```python
from build123d import *

# Parameters (mm, degrees)
SKETCH_1_W          = 60
SKETCH_1_H          = 17
EXTRUDE_1_DEPTH     = 1.2
CUT_EXTRUDE_1_REACH = 33.204
SKETCH_4_R          = 3.25
SKETCH_4_W          = 9.6
SKETCH_4_H          = 3.4
SKETCH_4_W_2        = 7
SKETCH_4_H_2        = 3.5
SKETCH_4_W_3        = 8
SKETCH_4_H_3        = 2.9
SKETCH_4_W_4        = 6.5
FILLET_2_R          = 1
CHAMFER_1_SIZE      = 0.6
SKETCH_5_W          = 1.5
SKETCH_5_H          = 8
EXTRUDE_2_DEPTH     = 1.2
SKETCH_6_W          = 28.5
SKETCH_6_H          = 1.6
EXTRUDE_3_DEPTH     = 4
FILLET_3_R          = 1
CHAMFER_2_SIZE      = 1
CHAMFER_4_SIZE      = 1
FILLET_4_R          = 2
CHAMFER_5_SIZE      = 0.4


with BuildPart() as part:
    # 草图1 → 凸台-拉伸1 (new body)
    with BuildSketch(Plane(origin=(0, 0, 0), x_dir=(1, 0, 0), z_dir=(0, 1, 0))):
        Rectangle(SKETCH_1_W, SKETCH_1_H)
    extrude(amount=EXTRUDE_1_DEPTH)

    # 草图4 → 切除-拉伸1 (cut, up to next)
    with BuildSketch(Plane(origin=(0, 1.2, 0), x_dir=(1, 0, 0), z_dir=(0, 1, 0)), mode=Mode.PRIVATE) as cut_extrude_1_sk1:
        with Locations(Location((22.298485985, 3.98318929, 0), (0, 0, 270))):
            Circle(SKETCH_4_R)
    cut_extrude_1_tool1 = extrude(cut_extrude_1_sk1.sketch, amount=-CUT_EXTRUDE_1_REACH, mode=Mode.PRIVATE) & part.part
    # 草图4 → 切除-拉伸1 (cut, up to next)
    with BuildSketch(Plane(origin=(0, 1.2, 0), x_dir=(1, 0, 0), z_dir=(0, 1, 0)), mode=Mode.PRIVATE) as cut_extrude_1_sk2:
        with Locations((-20.471722325, 2.6)):
            Rectangle(SKETCH_4_W, SKETCH_4_H)
    cut_extrude_1_tool2 = extrude(cut_extrude_1_sk2.sketch, amount=-CUT_EXTRUDE_1_REACH, mode=Mode.PRIVATE) & part.part
    # 草图4 → 切除-拉伸1 (cut, up to next)
    with BuildSketch(Plane(origin=(0, 1.2, 0), x_dir=(1, 0, 0), z_dir=(0, 1, 0)), mode=Mode.PRIVATE) as cut_extrude_1_sk3:
        with Locations((-5.682926277, 2.55)):
            Rectangle(SKETCH_4_W_2, SKETCH_4_H_2)
    cut_extrude_1_tool3 = extrude(cut_extrude_1_sk3.sketch, amount=-CUT_EXTRUDE_1_REACH, mode=Mode.PRIVATE) & part.part
    # 草图4 → 切除-拉伸1 (cut, up to next)
    with BuildSketch(Plane(origin=(0, 1.2, 0), x_dir=(1, 0, 0), z_dir=(0, 1, 0)), mode=Mode.PRIVATE) as cut_extrude_1_sk4:
        with Locations((7.788485985, 2.55)):
            Rectangle(SKETCH_4_W_2, SKETCH_4_H_2)
    cut_extrude_1_tool4 = extrude(cut_extrude_1_sk4.sketch, amount=-CUT_EXTRUDE_1_REACH, mode=Mode.PRIVATE) & part.part
    # 草图4 → 切除-拉伸1 (cut, up to next)
    with BuildSketch(Plane(origin=(0, 1.2, 0), x_dir=(1, 0, 0), z_dir=(0, 1, 0)), mode=Mode.PRIVATE) as cut_extrude_1_sk5:
        with Locations((21.05, -4.584803861)):
            Rectangle(SKETCH_4_W_3, SKETCH_4_H_3)
    cut_extrude_1_tool5 = extrude(cut_extrude_1_sk5.sketch, amount=-CUT_EXTRUDE_1_REACH, mode=Mode.PRIVATE) & part.part
    # 草图4 → 切除-拉伸1 (cut, up to next)
    with BuildSketch(Plane(origin=(0, 1.2, 0), x_dir=(1, 0, 0), z_dir=(0, 1, 0)), mode=Mode.PRIVATE) as cut_extrude_1_sk6:
        with Locations((-1.65, -4.884803861)):
            Rectangle(SKETCH_4_W_4, SKETCH_4_H_2)
    cut_extrude_1_tool6 = extrude(cut_extrude_1_sk6.sketch, amount=-CUT_EXTRUDE_1_REACH, mode=Mode.PRIVATE) & part.part
    # 草图4 → 切除-拉伸1 (cut, up to next)
    with BuildSketch(Plane(origin=(0, 1.2, 0), x_dir=(1, 0, 0), z_dir=(0, 1, 0)), mode=Mode.PRIVATE) as cut_extrude_1_sk7:
        with Locations((-10.15, -4.884803861)):
            Rectangle(SKETCH_4_W_4, SKETCH_4_H_2)
    cut_extrude_1_tool7 = extrude(cut_extrude_1_sk7.sketch, amount=-CUT_EXTRUDE_1_REACH, mode=Mode.PRIVATE) & part.part
    # 草图4 → 切除-拉伸1 (cut, up to next)
    with BuildSketch(Plane(origin=(0, 1.2, 0), x_dir=(1, 0, 0), z_dir=(0, 1, 0)), mode=Mode.PRIVATE) as cut_extrude_1_sk8:
        with Locations((-20.471722325, -4.834803861)):
            Rectangle(SKETCH_4_W, SKETCH_4_H)
    cut_extrude_1_tool8 = extrude(cut_extrude_1_sk8.sketch, amount=-CUT_EXTRUDE_1_REACH, mode=Mode.PRIVATE) & part.part
    add(cut_extrude_1_tool1.solids().sort_by_distance((22.298486, 1.2, -3.983189))[0], mode=Mode.SUBTRACT)
    add(cut_extrude_1_tool2.solids().sort_by_distance((-20.471722, 1.2, -2.6))[0], mode=Mode.SUBTRACT)
    add(cut_extrude_1_tool3.solids().sort_by_distance((-5.682926, 1.2, -2.55))[0], mode=Mode.SUBTRACT)
    add(cut_extrude_1_tool4.solids().sort_by_distance((7.788486, 1.2, -2.55))[0], mode=Mode.SUBTRACT)
    add(cut_extrude_1_tool5.solids().sort_by_distance((21.05, 1.2, 4.584804))[0], mode=Mode.SUBTRACT)
    add(cut_extrude_1_tool6.solids().sort_by_distance((-1.65, 1.2, 4.884804))[0], mode=Mode.SUBTRACT)
    add(cut_extrude_1_tool7.solids().sort_by_distance((-10.15, 1.2, 4.884804))[0], mode=Mode.SUBTRACT)
    add(cut_extrude_1_tool8.solids().sort_by_distance((-20.471722, 1.2, 4.834804))[0], mode=Mode.SUBTRACT)

    # 圆角2
    fillet_2_edges = [part.edges().sort_by_distance(p)[0] for p in [
        (-9.182926277, 0.6, -4.3),
        (-2.182926277, 0.6, -4.3),
        (4.288485985, 0.6, -4.3),
        (11.288485985, 0.6, -4.3),
        (17.05, 0.6, 6.034803861),
        (25.05, 0.6, 6.034803861),
        (-4.9, 0.6, 6.634803861),
        (-4.9, 0.6, 3.134803861),
        (1.6, 0.6, 3.134803861),
        (1.6, 0.6, 6.634803861),
        (-13.4, 0.6, 6.634803861),
        (-13.4, 0.6, 3.134803861),
        (-6.9, 0.6, 3.134803861),
        (-6.9, 0.6, 6.634803861),
        (-25.271722325, 0.6, 6.534803861),
        (-25.271722325, 0.6, 3.134803861),
        (-15.671722325, 0.6, 3.134803861),
        (-15.671722325, 0.6, 6.534803861),
        (-25.271722325, 0.6, -0.9),
        (-25.271722325, 0.6, -4.3),
        (-15.671722325, 0.6, -4.3),
        (-15.671722325, 0.6, -0.9),
    ]]
    fillet(fillet_2_edges, radius=FILLET_2_R)

    # 倒角1
    chamfer_1_edges = [part.edges().sort_by_distance(p)[0] for p in [
        (-9.182926277, 0.6, -0.8),
        (-2.182926277, 0.6, -0.8),
        (4.288485985, 0.6, -0.8),
        (11.288485985, 0.6, -0.8),
        (17.05, 0.6, 3.134803861),
        (25.05, 0.6, 3.134803861),
    ]]
    chamfer(chamfer_1_edges, length=CHAMFER_1_SIZE)

    # 草图5 → 凸台-拉伸2 (add)
    with BuildSketch(Plane.XZ):
        with Locations((-13.15891381, 0.61681071)):
            Rectangle(SKETCH_5_W, SKETCH_5_H)
        with Locations((13.84108619, 0.61681071)):
            Rectangle(SKETCH_5_W, SKETCH_5_H)
    extrude(amount=EXTRUDE_2_DEPTH)

    # 草图6 → 凸台-拉伸3 (add)
    with BuildSketch(Plane.XZ):
        with Locations((0.34108619, 1.3)):
            Rectangle(SKETCH_6_W, SKETCH_6_H)
    extrude(amount=EXTRUDE_3_DEPTH)

    # 圆角3
    fillet_3_edges = [part.edges().sort_by_distance(p)[0] for p in [
        (-13.90891381, -4, 1.3),
        (14.59108619, -4, 1.3),
    ]]
    fillet(fillet_3_edges, radius=FILLET_3_R)

    # 倒角2
    chamfer_2_edges = [part.edges().sort_by_distance(p)[0] for p in [
        (-13.15891381, -1.2, -3.38318929),
        (-13.15891381, -1.2, 4.61681071),
        (13.84108619, -1.2, -3.38318929),
        (13.84108619, -1.2, 4.61681071),
    ]]
    chamfer(chamfer_2_edges, length=CHAMFER_2_SIZE)

    # 倒角4
    chamfer_4_edges = [part.edges().sort_by_distance(p)[0] for p in [
        (-5.682926277, 0, -4.3),
        (-2.182926277, 0, -2.35),
        (7.788485985, 0, -4.3),
        (11.288485985, 0, -2.35),
        (21.05, 0, 6.034803861),
        (17.05, 0, 4.384803861),
        (-2.475819496, 0, -4.007106781),
        (-8.890033058, 0, -4.007106781),
        (4.581379204, 0, -4.007106781),
        (10.995592766, 0, -4.007106781),
        (24.757106781, 0, 5.741910642),
        (17.342893219, 0, 5.741910642),
        (-5.682926277, 0, -0.8),
        (-9.182926277, 0, -2.35),
        (7.788485985, 0, -0.8),
        (4.288485985, 0, -2.35),
        (21.05, 0, 3.134803861),
        (25.05, 0, 4.384803861),
        (-8.882926277, 0, -1.1),
        (-2.482926277, 0, -1.1),
        (4.588485985, 0, -1.1),
        (10.988485985, 0, -1.1),
        (17.35, 0, 3.434803861),
        (24.75, 0, 3.434803861),
    ]]
    chamfer(chamfer_4_edges, length=CHAMFER_4_SIZE)

    # 圆角4
    fillet_4_edges = [part.edges().sort_by_distance(p)[0] for p in [
        (30, 0.6, 8.5),
        (-30, 0.6, 8.5),
        (-30, 0.6, -8.5),
        (30, 0.6, -8.5),
    ]]
    fillet(fillet_4_edges, radius=FILLET_4_R)

    # 倒角5
    chamfer_5_edges = [part.edges().sort_by_distance(p)[0] for p in [
        (30, 0, 0),
        (0, 0, 8.5),
        (-30, 0, 0),
        (0, 0, -8.5),
        (-29.414213562, 0, -7.914213562),
        (-29.414213562, 0, 7.914213562),
        (29.414213562, 0, -7.914213562),
        (29.414213562, 0, 7.914213562),
    ]]
    chamfer(chamfer_5_edges, length=CHAMFER_5_SIZE)


solid = part.part
```
The listing builds one solid part. Answer for the finished solid, in the listing's coordinates (mm). A direction names the side the tool comes from. Coordinates: 2 decimals unless noted, no trailing zeros. Write each loop counter-clockwise with the first axis right and the second up, starting at its lowest first coordinate (ties: lowest second). Pieces come first, ordered by that corner, then holes. Notation, with made-up numbers: (-17, -10) - (10, -10) arc R22 cw to (10, 20) - close; hole circle Ø6 at (35, 1). An arc over 180 degrees is marked (long way). One line per item, written item: value.
1) For a pull along Z with two mould halves and no side action, classify faces 1 (the flat face through (-12.409, -1, 3)), 2 (the flat face through (-15.672, 1, -3)) as pulls with the +Z half, pulls with the -Z half, needs draft (parallel to the pull), parting line crosses it, or undercut.
Geometry check:
face 1: needs draft
face 2: undercut
2) A tool of negligible diameter and unlimited length cuts with its end or side. For faces 3 (the flat face through (16.56, 0.51, 4.38)), 4 (the cylindrical face through (1.3, 0.59, 6.35)), 5 (the flat face through (-13.4, 1, 5)), 6 (the cylindrical face through (-13.624, -3.699, 1.311)), 7 (the cylindrical face through (14.306, -3.699, 1.311)), from which of +Z, -Z, +X, -X, +Y, -Y can it reach the whole face along a straight path? Write none if from no direction.
Geometry check:
face 3: -Y
face 4: +Y, -Y
face 5: +Y
face 6: +Z, -Z, -X, -Y
face 7: +Z, -Z, +X, -Y
3) Consider line 1 along Z through (x, y) = (-18, 0.65); line 2 along Z through (x, y) = (23, 0.6); line 3 along Y through (x, z) = (-24.5, 3). Determine where each line is inside the solid, lowest interval first. Write a range as from..to.
Geometry check:
line 1: z = -8.5..-4.3, -0.9..3.13, 6.53..8.5
line 2: z = -8.5..-7.16, -0.81..2.73, 6.43..8.5
line 3: y = 0..1.2
4) Each of these flat-tipped pins is pushed along its axis until it touches: pin 1 Ø1.2 at (x, y) = (4.5, -2.5) entering from -Z; pin 2 Ø1.5 at (y, z) = (-1.5, 1.5) entering from +X; pin 3 Ø2 at (x, z) = (-4.5, -3.5) entering from -Y. Where does it stop, or does it pass through?
Geometry check:
pin 1: stops at z = 0.5
pin 2: stops at x = 14.59
pin 3: stops at y = 0.8
5) Find section B-B (z = 1.25). Give the vertices of the cut face in (x, y).
Geometry check:
outline: (-30, 0.4) - (-29.6, 0) - (-13.91, 0) - (-13.91, -3) arc R1 ccw to (-12.91, -4) - (13.59, -4) arc R1 ccw to (14.59, -3) - (14.59, 0) - (29.6, 0) - (30, 0.4) - (30, 1.2) - (-30, 1.2) - close
6) Find section A-A (x = 9). Give the vertices of the cut face in (y, z), and give its area (3 significant figures).
Geometry check:
outline: (-4, 0.5) - (0, 0.5) - (0, 0.2) - (1, -0.8) - (1.2, -0.8) - (1.2, 8.5) - (0.4, 8.5) - (0, 8.1) - (0, 2.1) - (-4, 2.1) - close; (0, -8.1) - (0.4, -8.5) - (1.2, -8.5) - (1.2, -4.3) - (1, -4.3) - (0, -5.3) - close
area: 21.4 mm2
